Geometry: final body of the model. Coordinates: model frame, mm. Face numbers are marked on the shaded views. A direction names the side the tool comes from. Coordinates: 2 decimals unless noted, no trailing zeros. Write each loop counter-clockwise with the first axis right and the second up, starting at its lowest first coordinate (ties: lowest second). Pieces come first, ordered by that corner, then holes. Notation, with made-up numbers: (5.5, -17.75) -> (59.5, -17.75) arc R26 ccw to (59.5, 7.25) -> close; hole circle Ø1 at (-32, 28). An arc over 180 degrees is marked (long way). One line per item, written item: value.
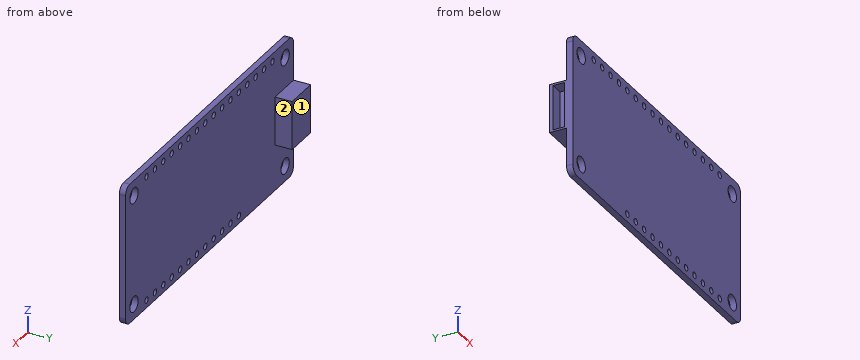
Autodesk Inventor part; units mm, degrees
ref_plane "YZ Plane" through (0, 0, 0) normal (1, 0, 0) x (0, 1, 0)
ref_plane "XZ Plane" through (0, 0, 0) normal (0, 1, 0) x (-1, 0, 0)
ref_plane "XY Plane" through (0, 0, 0) normal (0, 0, 1) x (1, 0, 0)
sketch "Sketch1" plane through (0, 0, 0) normal (0, 1, 0) x (-1, 0, 0)
  line L0 (0, 0) -> (-50.8, 0)
  line L1 (-50.8, 0) -> (-50.8, -22.86)
  line L2 (-50.8, -22.86) -> (0, -22.86)
  line L3 (0, -22.86) -> (0, 0)
  line L4 (0, 0) -> (-2.54, 0)
  line L5 (-2.54, 0) -> (-48.26, 0)
  line L6 (0, 0) -> (0, -2.54)
  line L7 (0, -2.54) -> (0, -20.32)
  dimension "d0" = 50.8
  dimension "d1" = 22.86
  dimension "d2" = 2.54
  dimension "d3" = 45.72
  dimension "d4" = 2.54
  dimension "d5" = 17.78
sketch "Sketch2" plane through (0, 0, 0) normal (0, 1, 0) x (-1, 0, 0)
  point P0 (0, 0)
sketch "Sketch3" plane through (0, 0, 0) normal (0, 1, 0) x (-1, 0, 0)
  line L0 (0, -1.27) -> (0, -1.27)
  line L1 (0, -2.504) -> (-2.54, -2.504)
  line L2 (-2.54, -2.504) -> (-2.54, 0)
  line L3 (0, -11.43) -> (-50.8, -11.43)
  circle A0 centre (-2.54, -2.504) radius 1.27
  circle A1 centre (-2.54, -20.356) radius 1.27
  line L4 (-25.4, 0) -> (-25.4, -22.86)
  circle A2 centre (-48.26, -2.504) radius 1.27
  circle A3 centre (-48.26, -20.356) radius 1.27
  line L5 (-1.27, 0) -> (-1.27, 0)
  arc A4 (0, -1.27) -> (-1.27, 0) centre (-1.27, -1.27) ccw
  arc A5 (-1.27, -22.86) -> (0, -21.59) centre (-1.27, -21.59) ccw
  arc A6 (-49.53, 0) -> (-50.8, -1.27) centre (-49.53, -1.27) ccw
  arc A7 (-50.8, -21.59) -> (-49.53, -22.86) centre (-49.53, -21.59) ccw
  line L6 (-25.4, -1.27) -> (-6.35, -1.27)
  line L7 (-25.4, -1.27) -> (-44.45, -1.27)
  circle A8 centre (-6.35, -1.27) radius 0.51
  line L8 (-6.35, -1.27) -> (-8.89, -1.27)
  line L9 (-6.35, -1.27) -> (-3.81, -1.27) construction
  circle A9 centre (-8.89, -1.27) radius 0.51
  circle A10 centre (-8.89, -1.27) radius 0.51
  circle A11 centre (-11.43, -1.27) radius 0.51
  circle A12 centre (-13.97, -1.27) radius 0.51
  circle A13 centre (-16.51, -1.27) radius 0.51
  circle A14 centre (-19.05, -1.27) radius 0.51
  circle A15 centre (-21.59, -1.27) radius 0.51
  circle A16 centre (-24.13, -1.27) radius 0.51
  circle A17 centre (-44.45, -1.27) radius 0.51
  circle A18 centre (-41.91, -1.27) radius 0.51
  circle A19 centre (-39.37, -1.27) radius 0.51
  circle A20 centre (-36.83, -1.27) radius 0.51
  circle A21 centre (-34.29, -1.27) radius 0.51
  circle A22 centre (-31.75, -1.27) radius 0.51
  circle A23 centre (-29.21, -1.27) radius 0.51
  circle A24 centre (-26.67, -1.27) radius 0.51
  circle A25 centre (-16.51, -21.59) radius 0.51
  circle A26 centre (-19.05, -21.59) radius 0.51
  circle A27 centre (-21.59, -21.59) radius 0.51
  circle A28 centre (-24.13, -21.59) radius 0.51
  circle A29 centre (-29.21, -21.59) radius 0.51
  circle A30 centre (-26.67, -21.59) radius 0.51
  circle A31 centre (-31.75, -21.59) radius 0.51
  circle A32 centre (-34.29, -21.59) radius 0.51
  circle A33 centre (-36.83, -21.59) radius 0.51
  circle A34 centre (-39.37, -21.59) radius 0.51
  circle A35 centre (-41.91, -21.59) radius 0.51
  circle A36 centre (-44.45, -21.59) radius 0.51
  line L10 (-1.27, -22.86) -> (-49.53, -22.86)
  line L11 (-50.8, -21.59) -> (-50.8, -1.27)
  line L12 (-49.53, 0) -> (-1.27, 0)
  line L13 (0, -1.27) -> (0, -21.59)
  point P0 (0, 0)
  dimension "d11" = 22.86
  dimension "d12" = 1.27
  dimension "d13" = 19.05
  dimension "d18" = 1.02
  dimension "d19" = 2.54
  dimension "d20" = 180
  dimension "d21" = 1.02
  dimension "d24" = 2.54
  dimension "d31" = 2.54
  dimension "d38" = 2.54
sketch "Sketch4" plane through (0, 0, 0) normal (0, 1, 0) x (-1, 0, 0)
  point P0 (0, 0)
extrude "Extrusion1" add sketch "Sketch3" along normal blind 1.016 contours L13 L3 L4 L12 L2 A0 L1 | L1 A0 L2 L12 A4 L13 | L13 A5 L10 L4 L3 | L4 L10 A7 L11 L3 | L3 L11 A6 L12 L4
sketch "Sketch5" plane through (0, 1.016, 0) normal (0, 1, 0) x (1, 0, 0)
  line L0 (0, 21.59) -> (0, 1.27)
  line L1 (0, 11.43) -> (0, 15.38)
  line L2 (0, 15.38) -> (5.6, 15.38)
  line L3 (5.6, 15.38) -> (5.6, 7.48)
  line L4 (5.6, 7.48) -> (0, 7.48)
  point P0 (0, 0)
  dimension "d46" = 3.95
  dimension "d49" = 5.6
  dimension "d50" = 7.9
extrude "Extrusion2" add sketch "Sketch5" along normal blind 2.8
sketch "Sketch6" plane through (5.6, 1.016, -7.48) normal (1, 0, 0) x (0, 0, -1)
  line L0 (0, 0) -> (0, 2.8)
  line L1 (7.9, 2.8) -> (0, 2.8)
  line L2 (7.9, 0) -> (7.9, 2.8)
  line L3 (-6.21, 0) -> (14.11, 0)
  point P0 (-7.48, -1.016)
sketch "Sketch7" plane through (0, 0, -21.59) normal (-1, 0, 0) x (0, 0, 1)
  line L0 (6.21, 3.816) -> (6.51, 3.816)
  line L1 (6.51, 3.216) -> (13.81, 3.216)
  line L2 (13.81, 3.216) -> (13.81, 1.316)
  line L3 (13.81, 1.316) -> (6.51, 1.316)
  line L4 (6.51, 1.316) -> (6.51, 3.216)
  point P0 (21.59, 0)
  dimension "d61" = 0.3
  dimension "d62" = 0.6
  dimension "d63" = 7.3
  dimension "d64" = 1.9
sketch "Sketch8" plane through (5.6, 1.016, -7.48) normal (1, 0, 0) x (0, 0, -1)
  point P0 (-7.48, -1.016)
extrude "Extrusion3" cut sketch "Sketch7" against normal blind 2.15
equation "\"BendRadius\" = Thickness"
equation "\"BendReliefWidth\" = Thickness"
equation "\"BendReliefDepth\" = 0.5 * Thickness"
equation "\"CornerReliefSize\" = 4 * Thickness"
equation "\"MinimumRemnant\" = 2 * Thickness"
equation "\"TransitionRadius\" = BendRadius"
equation "\"JacobiRadiusSize\" = Thickness"
equation "\"GapSize\" = Thickness"
properties part number "Adafruit Feather 32u4"
(1) First-contact query: pin 1 (0.9 mm diameter, centred on x = 44.45, z = -21.59, fed in from -Y); pin 2 (4 mm diameter, centred on x = 2.54, z = -2.504, fed in from +Y); pin 3 (1.4 mm diameter, centred on x = 1.5, y = 2.5, fed in from +Z); pin 4 (0.8 mm diameter, centred on y = 3, z = -11, fed in from +X). Flat tips, straight axial feed; report the tip coordinate or a pass-through.
Responses:
pin 1: passes through
pin 2: stops at y = 1.02
pin 3: stops at z = -7.48
pin 4: stops at x = 5.6
(2) Section D-D (x = 18). Return the cut outline in (y, z).
Responses:
outline: (0, -22.86) -> (1.02, -22.86) -> (1.02, 0) -> (0, 0) -> close
(3) Section A-A (x = 39.37). Return the cut outline in (y, z), then the cut area to 3 significant figures.
Responses:
outline: (0, -22.86) -> (1.02, -22.86) -> (1.02, -22.1) -> (0, -22.1) -> close; (0, -21.08) -> (1.02, -21.08) -> (1.02, -1.78) -> (0, -1.78) -> close; (0, -0.76) -> (1.02, -0.76) -> (1.02, 0) -> (0, 0) -> close
area: 21.2 mm2
(4) Line query: line 1 (Z direction, x = 31.75, y = 0.65); line 2 (Z direction, x = 2.54, y = 0.5); line 3 (X direction, y = 1.2, z = -11.75). Output: solid intervals per line, ascending. Write a range as [from, to].
Responses:
line 1: z = [-22.86, -22.1], [-21.08, -1.78], [-0.76, 0]
line 2: z = [-22.86, -21.63], [-19.09, -3.77], [-1.23, 0]
line 3: x = [0, 5.6]
(5) Section C-C (z = -6). Return the cut outline in (x, y), then the cut area to 3 significant figures.
Responses:
outline: (0, 0) -> (50.8, 0) -> (50.8, 1.02) -> (0, 1.02) -> close
area: 51.6 mm2
(6) Section B-B (y = 1.95). Return the cut outline in (x, z).
Responses:
outline: (0, -15.38) -> (5.6, -15.38) -> (5.6, -7.48) -> (0, -7.48) -> (0, -7.78) -> (2.15, -7.78) -> (2.15, -15.08) -> (0, -15.08) -> close
(7) Reachability of the marked faces 1 and 2 from +Z, -Z, +X, -X, +Y, -Y: full face, straight path, thin tool, end or side. Return the list, or none.
Responses:
face 1: +Z, -Z, +X, -X, +Y
face 2: +Z, -Z, +X, +Y
